The listing builds one solid part. Answer for the finished solid, in the listing's coordinates (mm). A direction names the side the tool comes from. Round coordinates to 2 decimals unless told otherwise and drop trailing zeros. Write each loop counter-clockwise with the first axis right and the second up, starting at its lowest first coordinate (ties: lowest second). Pieces come first, ordered by that corner, then holes.
(1) Each of these flat-tipped pins is pushed along its axis until it touches: pin 1 Ø1.1 at (x, y) = (7.5, 0) entering from -Z; pin 2 Ø5 at (y, z) = (-7, 5) entering from -X; pin 3 Ø10 at (y, z) = (7.5, 17) entering from -X; pin 4 Ø3 at (x, y) = (3, 1.5) entering from -Z. Where does it stop, or does it pass through?
(2) A cutting plane is placed at A-A, the plane x = 0. Give the vertices of the cut face in (y, z).
(3) A cutting plane is placed at C-C, the plane z = 13.5. Give the vertices of the cut face in (x, y), and give its area (3 significant figures).
(4) Find the intervals of material crossed by probe 1 along Y at (x, z) = (2.25, 3); probe 2 along X at (y, z) = (4, 1.25); probe 3 along Y at (x, z) = (0, 9.5), in increasing order.
(5) A cutting plane is placed at D-D, the plane y = -1.25. Give the vertices of the cut face in (x, z).
(6) A cutting plane is placed at B-B, the plane z = 18.5. Give the vertices of the cut face in (x, y), and give its area (3 significant figures).
(7) For faces 1 (the face through (-8.2, 0, 7.9)), 2 (the face through (0, 9, 10)), 3 (the face through (-7.158, -4.056, 14.93)), 4 (the face through (8, 4, 10)), determine the directions among +Z, -Z, +X, -X, +Y, -Y from which every point of the face is accessible in a straight line to the end or side of a thin tool.
(8) The mould has two halves that part along Y. Classify faces 5 (the face through (4, -4, 0)), 6 (the face through (6.8, 0, 7.9)), 7 (the face through (0, -8.227, 15)): +Y half, -Y half, draft (parallel to the pull), parting line (faces both ways), or undercut.
from build123d import *

# Parameters (mm, degrees)
F0_R     = 9.5
F0_R_2   = 0.7
F0_R_3   = 5.5
F1_DEPTH = 10
F2_DEPTH = 5
F3_R     = 0.7
F3_R_2   = 5.5
F4_DEPTH = 6
F5_R     = 0.7
F5_R_2   = 5.5
F6_DEPTH = 4


with BuildPart() as f1:
    # F0 (on Top) → F1 (new body)
    with BuildSketch(Plane.XY):
        Circle(F0_R)
        with Locations((-7.5, 0)):
            Circle(F0_R_2, mode=Mode.SUBTRACT)
        Circle(F0_R_3, mode=Mode.SUBTRACT)
        with Locations((7.5, 0)):
            Circle(F0_R_2, mode=Mode.SUBTRACT)
    extrude(amount=F1_DEPTH)

    # F0 (on Top) → F2 (cut)
    with BuildSketch(Plane.XY):
        Circle(F0_R_3)
    extrude(amount=F2_DEPTH, mode=Mode.SUBTRACT)

    # F3 (on face) → F4 (join)
    with BuildSketch(Plane.XY.offset(10)):
        Polygon((4.75, -8.227241336), (9.5, 0), (4.75, 8.227241336), (-4.75, 8.227241336), (-9.5, 0), (-4.75, -8.227241336), align=None)
        with Locations((-7.5, 0)):
            Circle(F3_R, mode=Mode.SUBTRACT)
        Circle(F3_R_2, mode=Mode.SUBTRACT)
        with Locations((7.5, 0)):
            Circle(F3_R, mode=Mode.SUBTRACT)
    extrude(amount=F4_DEPTH)

    # F5 (on face) → F6 (join)
    with BuildSketch(Plane.XY.offset(16)):
        Polygon((4.75, -8.227241336), (9.5, 0), (4.75, 8.227241336), (-4.75, 8.227241336), (-9.5, 0), (-4.75, -8.227241336), align=None)
        with Locations((-7.5, 0)):
            Circle(F5_R, mode=Mode.SUBTRACT)
        Circle(F5_R_2, mode=Mode.SUBTRACT)
        with Locations((7.5, 0)):
            Circle(F5_R, mode=Mode.SUBTRACT)
        with Locations((-7.5, 0)):
            Circle(F5_R)
        with Locations((7.5, 0)):
            Circle(F5_R)
    extrude(amount=F6_DEPTH)


solid = f1.part
Solutions:
1. pin 1: stops at z = 16
1. pin 2: stops at x = -8.37
1. pin 3: stops at x = -8.06
1. pin 4: passes through
2. outline: (-9.5, 0) - (-5.5, 0) - (-5.5, 20) - (-8.23, 20) - (-8.23, 10) - (-9.5, 10) - close; (5.5, 0) - (9.5, 0) - (9.5, 10) - (8.23, 10) - (8.23, 20) - (5.5, 20) - close
3. outline: (-9.5, 0) - (-4.75, -8.23) - (4.75, -8.23) - (9.5, 0) - (4.75, 8.23) - (-4.75, 8.23) - close; hole circle Ø1.4 at (-7.5, 0); hole circle Ø11 at (0, 0); hole circle Ø1.4 at (7.5, 0)
3. area: 136 mm2
4. probe 1: y = -9.23 to -5.02, 5.02 to 9.23
4. probe 2: x = -8.62 to -3.77, 3.77 to 8.62
4. probe 3: y = -9.5 to -5.5, 5.5 to 9.5
5. outline: (-9.42, 0) - (-5.36, 0) - (-5.36, 20) - (-8.78, 20) - (-8.78, 10) - (-9.42, 10) - close; (5.36, 0) - (9.42, 0) - (9.42, 10) - (8.78, 10) - (8.78, 20) - (5.36, 20) - close
6. outline: (-9.5, 0) - (-4.75, -8.23) - (4.75, -8.23) - (9.5, 0) - (4.75, 8.23) - (-4.75, 8.23) - close; hole circle Ø11 at (0, 0)
6. area: 139 mm2
7. face 1: -Z
7. face 2: +Z, +X, -X, +Y
7. face 3: +Z, -X, -Y
7. face 4: +Z, +X, +Y
8. face 5: draft
8. face 6: undercut
8. face 7: -Y half
